```python
from build123d import *

# Parameters (mm, degrees)
F0_W     = 44.45
F0_H     = 222.25
F1_DEPTH = 12.7


with BuildPart() as f1:
    # F0 (on Top) → F1 (new body)
    with BuildSketch(Plane.XY):
        with BuildLine():
            Line((-227.80625, 254), (-227.80625, -31.75))
            Line((-227.80625, -31.75), (-183.35625, -31.75))
            ThreePointArc((-183.35625, -31.75), (-173.83125, -22.225), (-164.30625, -31.75))
            Line((-164.30625, -31.75), (-138.1125, -31.75))
            ThreePointArc((-138.1125, -31.75), (-128.5875, -22.225), (-119.0625, -31.75))
            Line((-119.0625, -31.75), (-92.86875, -31.75))
            ThreePointArc((-92.86875, -31.75), (-83.34375, -22.225), (-73.81875, -31.75))
            Line((-73.81875, -31.75), (-47.625, -31.75))
            ThreePointArc((-47.625, -31.75), (-38.1, -22.225), (-28.575, -31.75))
            Line((-28.575, -31.75), (-2.38125, -31.75))
            ThreePointArc((-2.38125, -31.75), (0.408558, -25.014808), (7.14375, -22.225))
            Line((7.14375, -22.225), (7.14375, 254))
            Line((7.14375, 254), (-227.80625, 254))
        make_face()
        with Locations((-205.58125, -142.875)):
            Rectangle(F0_W, F0_H)
        with Locations((219.86875, -142.875)):
            Rectangle(F0_W, F0_H)
        with BuildLine():
            ThreePointArc((178.59375, -31.75), (188.11875, -22.225), (197.64375, -31.75))
            Line((197.64375, -31.75), (242.09375, -31.75))
            Line((242.09375, -31.75), (242.09375, 254))
            Line((242.09375, 254), (7.14375, 254))
            Line((7.14375, 254), (7.14375, -22.225))
            ThreePointArc((7.14375, -22.225), (13.878942, -25.014808), (16.66875, -31.75))
            Line((16.66875, -31.75), (42.8625, -31.75))
            ThreePointArc((42.8625, -31.75), (52.3875, -22.225), (61.9125, -31.75))
            Line((61.9125, -31.75), (88.10625, -31.75))
            ThreePointArc((88.10625, -31.75), (97.63125, -22.225), (107.15625, -31.75))
            Line((107.15625, -31.75), (133.35, -31.75))
            ThreePointArc((133.35, -31.75), (142.875, -22.225), (152.4, -31.75))
            Line((152.4, -31.75), (165.496875, -31.75))
            Line((165.496875, -31.75), (178.59375, -31.75))
        make_face()
        with BuildLine():
            Line((173.434375, -57.15), (178.59375, -31.75))
            Line((178.59375, -31.75), (165.496875, -31.75))
            Line((165.496875, -31.75), (165.496875, -49.2125))
            ThreePointArc((165.496875, -49.2125), (171.109535, -51.53734), (173.434375, -57.15))
        make_face()
        with BuildLine():
            Line((165.496875, -49.2125), (165.496875, -31.75))
            Line((165.496875, -31.75), (152.4, -31.75))
            Line((152.4, -31.75), (157.559375, -57.15))
            ThreePointArc((157.559375, -57.15), (159.884215, -51.53734), (165.496875, -49.2125))
        make_face()
        with BuildLine():
            ThreePointArc((157.559375, -57.15), (165.496875, -65.0875), (173.434375, -57.15))
            ThreePointArc((173.434375, -57.15), (171.109535, -51.53734), (165.496875, -49.2125))
            ThreePointArc((165.496875, -49.2125), (159.884215, -51.53734), (157.559375, -57.15))
        make_face()
        with BuildLine():
            Line((128.190625, -57.15), (133.35, -31.75))
            Line((133.35, -31.75), (107.15625, -31.75))
            Line((107.15625, -31.75), (112.315625, -57.15))
            ThreePointArc((112.315625, -57.15), (120.253125, -49.2125), (128.190625, -57.15))
        make_face()
        with BuildLine():
            ThreePointArc((112.315625, -57.15), (120.253125, -65.0875), (128.190625, -57.15))
            ThreePointArc((128.190625, -57.15), (120.253125, -49.2125), (112.315625, -57.15))
        make_face()
        with BuildLine():
            Line((88.10625, -31.75), (61.9125, -31.75))
            Line((61.9125, -31.75), (67.071875, -57.15))
            ThreePointArc((67.071875, -57.15), (75.009375, -49.2125), (82.946875, -57.15))
            Line((82.946875, -57.15), (88.10625, -31.75))
        make_face()
        with BuildLine():
            ThreePointArc((82.946875, -57.15), (75.009375, -49.2125), (67.071875, -57.15))
            ThreePointArc((67.071875, -57.15), (75.009375, -65.0875), (82.946875, -57.15))
        make_face()
        with BuildLine():
            Line((42.8625, -31.75), (16.66875, -31.75))
            Line((16.66875, -31.75), (21.828125, -57.15))
            ThreePointArc((21.828125, -57.15), (29.765625, -49.2125), (37.703125, -57.15))
            Line((37.703125, -57.15), (42.8625, -31.75))
        make_face()
        with BuildLine():
            ThreePointArc((37.703125, -57.15), (29.765625, -49.2125), (21.828125, -57.15))
            ThreePointArc((21.828125, -57.15), (29.765625, -65.0875), (37.703125, -57.15))
        make_face()
        with BuildLine():
            Line((-7.540625, -57.15), (-2.38125, -31.75))
            Line((-2.38125, -31.75), (-28.575, -31.75))
            Line((-28.575, -31.75), (-23.415625, -57.15))
            ThreePointArc((-23.415625, -57.15), (-15.478125, -49.2125), (-7.540625, -57.15))
        make_face()
        with BuildLine():
            ThreePointArc((-23.415625, -57.15), (-15.478125, -65.0875), (-7.540625, -57.15))
            ThreePointArc((-7.540625, -57.15), (-15.478125, -49.2125), (-23.415625, -57.15))
        make_face()
        with BuildLine():
            Line((-47.625, -31.75), (-73.81875, -31.75))
            Line((-73.81875, -31.75), (-68.659375, -57.15))
            ThreePointArc((-68.659375, -57.15), (-60.721875, -49.2125), (-52.784375, -57.15))
            Line((-52.784375, -57.15), (-47.625, -31.75))
        make_face()
        with BuildLine():
            ThreePointArc((-52.784375, -57.15), (-60.721875, -49.2125), (-68.659375, -57.15))
            ThreePointArc((-68.659375, -57.15), (-60.721875, -65.0875), (-52.784375, -57.15))
        make_face()
        with BuildLine():
            Line((-92.86875, -31.75), (-119.0625, -31.75))
            Line((-119.0625, -31.75), (-113.903125, -57.15))
            ThreePointArc((-113.903125, -57.15), (-105.965625, -49.2125), (-98.028125, -57.15))
            Line((-98.028125, -57.15), (-92.86875, -31.75))
        make_face()
        with BuildLine():
            ThreePointArc((-98.028125, -57.15), (-105.965625, -49.2125), (-113.903125, -57.15))
            ThreePointArc((-113.903125, -57.15), (-105.965625, -65.0875), (-98.028125, -57.15))
        make_face()
        with BuildLine():
            Line((-138.1125, -31.75), (-164.30625, -31.75))
            Line((-164.30625, -31.75), (-159.146875, -57.15))
            ThreePointArc((-159.146875, -57.15), (-151.209375, -49.2125), (-143.271875, -57.15))
            Line((-143.271875, -57.15), (-138.1125, -31.75))
        make_face()
        with BuildLine():
            ThreePointArc((-143.271875, -57.15), (-151.209375, -49.2125), (-159.146875, -57.15))
            ThreePointArc((-159.146875, -57.15), (-151.209375, -65.0875), (-143.271875, -57.15))
        make_face()
    extrude(amount=F1_DEPTH)


solid = f1.part
```
Read the model definition and answer for the solid it produces. Units are mm, in the model's axes. A direction names the side the tool comes from. Give positions to 0.01 mm unless a question says otherwise; leave off trailing zeros. Write each loop counter-clockwise with the first axis right and the second up, starting at its lowest first coordinate (ties: lowest second). Pieces come first, ordered by that corner, then holes. Notation, with made-up numbers: (-37, 41) -> (5, 41) arc R22 cw to (5, 70) -> close; hole circle Ø11 at (-35, 22.5). An arc over 180 degrees is marked (long way). Answer as a JSON object with one key per item and string values.
1) Section A-A on y = -168.5 is taken. Write down the section's boundary in (x, z), then the cut area to 3 significant figures.
Findings below:
{"outline": "(-227.81, 0) -> (-183.36, 0) -> (-183.36, 12.7) -> (-227.81, 12.7) -> close; (197.64, 0) -> (242.09, 0) -> (242.09, 12.7) -> (197.64, 12.7) -> close", "area": "1,130 mm^2"}
2) A tool of negligible diameter and unlimited length cuts with its end or side. For faces 4 (the flat face through (-206, -254, 6)), 5 (the flat face through (40.247, -44.628, 6.261)), from which of +Z, -Z, +X, -X, +Y, -Y can it reach the whole face along a straight path? Write none if from no direction.
Findings below:
{"face 4": "+Z, -Z, +X, -X, -Y", "face 5": "+Z, -Z, -Y"}
3) For a pull along X with two mould halves and no side action, classify faces 1 (the flat face through (-227.806, 4, 6)), 2 (the flat face through (-183.356, -144, 6)), 3 (the flat face through (10, 254, 6)) as pulls with the +X half, pulls with the -X half, needs draft (parallel to the pull), parting line crosses it, or undercut.
Findings below:
{"face 1": "pulls with the -X half", "face 2": "undercut", "face 3": "needs draft"}
4) Section B-B on x = -38.1 is taken. Write down the section's boundary in (y, z) (3 decimals), then the cut area to 3 significant figures.
Findings below:
{"outline": "(-22.225, 0) -> (254, 0) -> (254, 12.7) -> (-22.225, 12.7) -> close", "area": "3,510 mm^2"}
5) A flat-ended cylindrical pin translates along its axis: pin 1 Ø1 at (x, z) = (-89.5, 9) entering from -Y. Find the tip coordinate at first contact, or state that the pin passes through.
Findings below:
{"pin 1": "stops at y = -24.94"}
6) Straight lines are drawn through the part: probe 1 along X at (y, z) = (-117, 4.25); probe 2 along Y at (x, z) = (69, 11); probe 3 along Y at (x, z) = (-148.5, 7.5). For each, find the intervals that lie inside material, in ascending order. Write a range as from..to.
Findings below:
{"probe 1": "x = -227.81..-183.36, 197.64..242.09", "probe 2": "y = -62.34..254", "probe 3": "y = -64.61..254"}
7) Section C-C on x = -105.5 is taken. Write down the section's boundary in (y, z).
Findings below:
{"outline": "(-65.07, 0) -> (254, 0) -> (254, 12.7) -> (-65.07, 12.7) -> close"}
